Source: CAD feature listing. Evaluate the final solid. Frame: model axes, mm. Face numbers are marked on the shaded views. A direction names the side the tool comes from. Round coordinates to 2 decimals unless told otherwise and drop trailing zeros. Write each loop counter-clockwise with the first axis right and the second up, starting at its lowest first coordinate (ties: lowest second). Pieces come first, ordered by that corner, then holes.
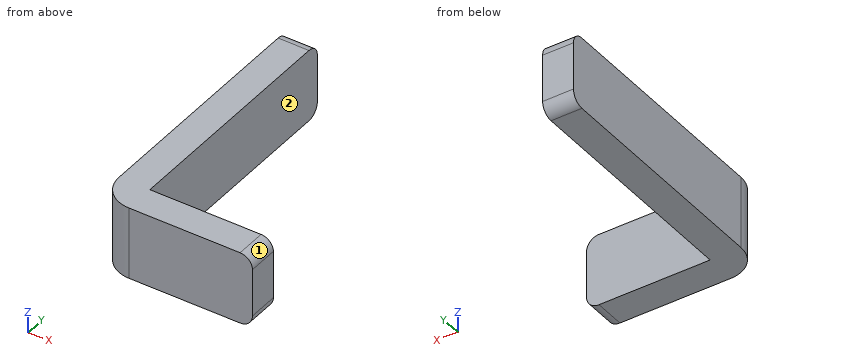
from build123d import *

# Parameters (mm, degrees)
SKETCH1_W           = 25
SKETCH1_H           = 11.704143749
BOSS_EXTRUDE1_DEPTH = 5
SKETCH2_W           = 5
SKETCH2_H           = 11.704143749
BOSS_EXTRUDE2_DEPTH = 40
FILLET1_R           = 5
FILLET2_R           = 2


with BuildPart() as part:
    # Sketch1 → Boss-Extrude1 (new body)
    with BuildSketch(Plane(origin=(0, 0, 0), x_dir=(1, 0, 0), z_dir=(0, 1, 0))):
        with Locations((12.5, 5.852071874)):
            Rectangle(SKETCH1_W, SKETCH1_H)
    extrude(amount=BOSS_EXTRUDE1_DEPTH)

    # Sketch2 → Boss-Extrude2 (add)
    with BuildSketch(Plane(origin=(0, 5, 0), x_dir=(1, 0, 0), z_dir=(0, 1, 0))):
        with Locations((2.5, 5.852071874)):
            Rectangle(SKETCH2_W, SKETCH2_H)
    extrude(amount=BOSS_EXTRUDE2_DEPTH)

    # Fillet1
    fillet1_edges = [part.edges().sort_by_distance(p)[0] for p in [
        (0, 0, -5.852071875),
    ]]
    fillet(fillet1_edges, radius=FILLET1_R)

    # Fillet2
    fillet2_edges = [part.edges().sort_by_distance(p)[0] for p in [
        (2.5, 45, 0),
        (2.5, 45, -11.704143749),
        (25, 2.5, -11.704143749),
        (25, 2.5, 0),
    ]]
    fillet(fillet2_edges, radius=FILLET2_R)


solid = part.part
1) Section query B-B on x = 20.5. Return the cut outline in (y, z), then the cut area to 3 significant figures.
Taken from the geometry:
outline: (0, -11.7) - (5, -11.7) - (5, 0) - (0, 0) - close
area: 58.5 mm2
2) Section query A-A on z = -2.75. Return the cut outline in (x, y).
Taken from the geometry:
outline: (0, 5) arc R5 ccw to (5, 0) - (25, 0) - (25, 5) - (5, 5) - (5, 45) - (0, 45) - close
3) Section query D-D on z = -10.5. Return the cut outline in (x, y), then the cut area to 3 significant figures.
Taken from the geometry:
outline: (0, 5) arc R5 ccw to (5, 0) - (24.83, 0) - (24.83, 5) - (5, 5) - (5, 44.83) - (0, 44.83) - close
area: 318 mm2
4) Contact query for flat-ended pins moving along their axis: P1, Ø1, axis at x = 3, z = -3, coming from the -Y side; P2, Ø6, axis at x = 17.5, z = -7, coming from the +Y side. Output: stop coordinate, or through.
Taken from the geometry:
P1: stops at y = 0.23
P2: stops at y = 5
5) Reachability of the marked faces 1 and 2 from +Z, -Z, +X, -X, +Y, -Y: full face, straight path, thin tool, end or side. Return the list, or none.
Taken from the geometry:
face 1: +Z, +X, +Y, -Y
face 2: +Z, -Z, +X, +Y
6) Material intervals for line 1 (Y direction, x = 16.75, z = -10.75); line 2 (X direction, y = 2.5, z = -4.5), sorted ascending.
Taken from the geometry:
line 1: y = 0 to 5
line 2: x = 0.67 to 25
